Work out the finished part from the listing and answer in its coordinate system (mm). Face numbers are marked on the shaded views. A direction names the side the tool comes from. Give positions to 0.01 mm unless a question says otherwise; leave off trailing zeros. Write each loop counter-clockwise with the first axis right and the second up, starting at its lowest first coordinate (ties: lowest second). Pieces come first, ordered by that corner, then holes. Notation, with made-up numbers: (-14.75, -39) -> (32.25, -39) arc R28 ccw to (32.25, -9) -> close; hole circle Ø11 at (-21, -32). An arc over 180 degrees is marked (long way). Use a Markdown table: item, result. Add a question column.
Q1. Each of these flat-tipped pins is pushed along its axis until it touches: pin 1 Ø2.5 at (y, z) = (0.5, 13) entering from -X; pin 2 Ø7 at (y, z) = (2, 17.5) entering from -X; pin 3 Ø1 at (y, z) = (3.5, 9.5) entering from -X. Where does it stop, or does it pass through?
Q2. Consider line 1 (Y direction, x = -0.75, z = 12.25); line 2 (Y direction, x = -4, z = 10); line 3 (X direction, y = 4.5, z = 23.75). Determine where each line is inside the solid, lowest interval first.
Q3. Section A-A, the plane x = 9.25 is taken. Give the vertices of the cut face in (y, z), plus the area to 3 significant figures.
Q4. Section B-B, the plane z = 5.75 is taken. State how many separate pieces and enclosed holes the cut face has, plus the area to 3 significant figures.
Q5. For a pull along X with two mould halves and no side action, classify the marked faces 1, 2 and 3 as pulls with the +X half, pulls with the -X half, needs draft (parallel to the pull), parting line crosses it, or undercut.
Q6. For the marked faces 4, 5 and 6, determine the directions among +Z, -Z, +X, -X, +Y, -Y from which every point of the face is accessible in a straight line to the end or side of a thin tool.
from build123d import *

# Parameters (mm, degrees)
EXTRUDE1_DEPTH = 25.4


with BuildPart() as part:
    # Sketch1 → Extrude1 (new body)
    with BuildSketch(Plane.XY):
        with BuildLine():
            Line((-8.268033791, 7.446247994), (-5.358427067, 4.536641271))
            ThreePointArc((-5.358427067, 4.536641271), (-4.478329805, 3.219482637), (-4.169280745, 1.665788092))
            Line((-4.169280745, 1.665788092), (-4.169280745, 0))
            Line((-4.169280745, 0), (-4.169280745, -1.665788092))
            ThreePointArc((-4.169280745, -1.665788092), (-4.478329805, -3.219482637), (-5.358427067, -4.536641271))
            Line((-5.358427067, -4.536641271), (-8.268033791, -7.446247994))
            ThreePointArc((-8.268033791, -7.446247994), (-9.379617585, -7.667355758), (-10.009279225, -6.72500052))
            Line((-10.009279225, -6.72500052), (-10.009279225, -4.25999656))
            ThreePointArc((-10.009279225, -4.25999656), (-10.308029711, -3.538749086), (-11.029277185, -3.2399986))
            Line((-11.029277185, -3.2399986), (-11.23000167, -3.2399986))
            ThreePointArc((-11.23000167, -3.2399986), (-11.937549497, -3.525304849), (-12.249277285, -4.221616108))
            Line((-12.249277285, -4.221616108), (-12.49887312, -10.850171322))
            ThreePointArc((-12.49887312, -10.850171322), (-12.055256326, -12.012943733), (-10.90999977, -12.49999913))
            Line((-10.90999977, -12.49999913), (0, -12.49999913))
            Line((0, -12.49999913), (10.90999977, -12.49999913))
            ThreePointArc((10.90999977, -12.49999913), (12.0342991, -12.0342991), (12.49999913, -10.90999977))
            Line((12.49999913, -10.90999977), (12.49999913, 10.90999977))
            ThreePointArc((12.49999913, 10.90999977), (12.0342991, 12.0342991), (10.90999977, 12.49999913))
            Line((10.90999977, 12.49999913), (0, 12.49999913))
            Line((0, 12.49999913), (-10.90999977, 12.49999913))
            ThreePointArc((-10.90999977, 12.49999913), (-12.055256326, 12.012943733), (-12.49887312, 10.850171322))
            Line((-12.49887312, 10.850171322), (-12.249277285, 4.221616108))
            ThreePointArc((-12.249277285, 4.221616108), (-11.937549497, 3.525304849), (-11.23000167, 3.2399986))
            Line((-11.23000167, 3.2399986), (-11.029277185, 3.2399986))
            ThreePointArc((-11.029277185, 3.2399986), (-10.308029711, 3.538749086), (-10.009279225, 4.25999656))
            Line((-10.009279225, 4.25999656), (-10.009279225, 6.72500052))
            ThreePointArc((-10.009279225, 6.72500052), (-9.379617585, 7.667355758), (-8.268033791, 7.446247994))
        make_face()
        with BuildLine():
            Line((-7.539973637, 8.825029193), (-4.084091296, 5.369146852))
            ThreePointArc((-4.084091296, 5.369146852), (-2.766932662, 4.48904959), (-1.213238118, 4.18000053))
            Line((-1.213238118, 4.18000053), (0, 4.18000053))
            Line((0, 4.18000053), (1.439511835, 4.18000053))
            ThreePointArc((1.439511835, 4.18000053), (2.993206379, 4.48904959), (4.310365013, 5.369146852))
            Line((4.310365013, 5.369146852), (7.493110816, 8.551892654))
            ThreePointArc((7.493110816, 8.551892654), (7.679535009, 9.489110364), (6.8850002, 10.02000155))
            Line((6.8850002, 10.02000155), (0, 10.02000155))
            Line((0, 10.02000155), (-7.04499988, 10.02000155))
            ThreePointArc((-7.04499988, 10.02000155), (-7.691714259, 9.587880817), (-7.539973637, 8.825029193))
        make_face(mode=Mode.SUBTRACT)
        with BuildLine():
            Line((0, -10.02000155), (-7.04499988, -10.02000155))
            ThreePointArc((-7.04499988, -10.02000155), (-7.691714259, -9.587880817), (-7.539973637, -8.825029193))
            Line((-7.539973637, -8.825029193), (-4.084091296, -5.369146852))
            ThreePointArc((-4.084091296, -5.369146852), (-2.766932662, -4.48904959), (-1.213238118, -4.18000053))
            Line((-1.213238118, -4.18000053), (0, -4.18000053))
            Line((0, -4.18000053), (1.439511835, -4.18000053))
            ThreePointArc((1.439511835, -4.18000053), (2.993206379, -4.48904959), (4.310365013, -5.369146852))
            Line((4.310365013, -5.369146852), (7.493110816, -8.551892654))
            ThreePointArc((7.493110816, -8.551892654), (7.679535009, -9.489110364), (6.8850002, -10.02000155))
            Line((6.8850002, -10.02000155), (0, -10.02000155))
        make_face(mode=Mode.SUBTRACT)
        with BuildLine():
            Line((8.551892654, 7.493110816), (5.369146852, 4.310365013))
            ThreePointArc((5.369146852, 4.310365013), (4.48904959, 2.993206379), (4.18000053, 1.439511835))
            Line((4.18000053, 1.439511835), (4.18000053, -1.439511835))
            ThreePointArc((4.18000053, -1.439511835), (4.48904959, -2.993206379), (5.369146852, -4.310365013))
            Line((5.369146852, -4.310365013), (8.551892654, -7.493110816))
            ThreePointArc((8.551892654, -7.493110816), (9.489110364, -7.679535009), (10.02000155, -6.8850002))
            Line((10.02000155, -6.8850002), (10.02000155, 6.8850002))
            ThreePointArc((10.02000155, 6.8850002), (9.489110364, 7.679535009), (8.551892654, 7.493110816))
        make_face(mode=Mode.SUBTRACT)
        with BuildLine():
            ThreePointArc((0, 2.55499997), (-1.806657805, 1.806657805), (-2.55499997, 0))
            ThreePointArc((-2.55499997, 0), (-1.806657805, -1.806657805), (0, -2.55499997))
            ThreePointArc((0, -2.55499997), (1.806657805, -1.806657805), (2.55499997, 0))
            ThreePointArc((2.55499997, 0), (1.806657805, 1.806657805), (0, 2.55499997))
        make_face(mode=Mode.SUBTRACT)
    extrude(amount=EXTRUDE1_DEPTH)


solid = part.part
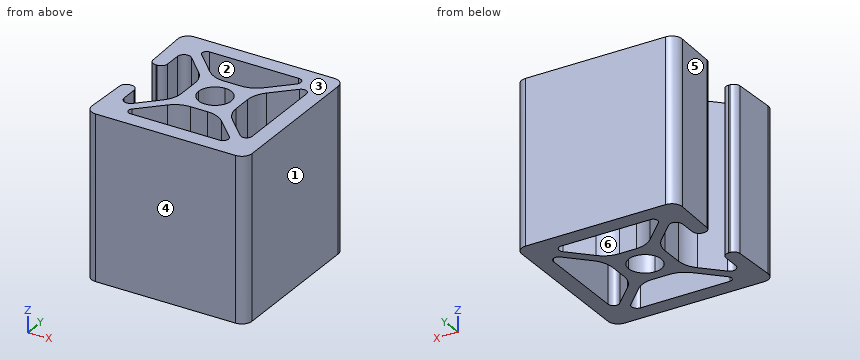
Result set:
| question | item | result |
|---|---|---|
| 1 | pin 1 | stops at x = -4.17 |
| 1 | pin 2 | stops at x = -12.3 |
| 1 | pin 3 | stops at x = -12.22 |
| 2 | line 1 | y = -12.5 to -10.02, -4.18 to -2.44, 2.44 to 4.18, 10.02 to 12.5 |
| 2 | line 2 | y = -12.5 to -10.02, -5.29 to 5.29, 10.02 to 12.5 |
| 2 | line 3 | x = -12.26 to -10.01, -5.32 to -2.79, 3.02 to 5.56, 10.02 to 12.5 |
| 3 | outline | (-12.5, 0) -> (-7.74, 0) -> (-7.74, 25.4) -> (-12.5, 25.4) -> close; (7.74, 0) -> (12.5, 0) -> (12.5, 25.4) -> (7.74, 25.4) -> close |
| 3 | area | 242 mm2 |
| 4 | separate pieces | 1 |
| 4 | enclosed holes | 4 |
| 4 | area | 311 mm2 |
| 5 | face 1 | pulls with the +X half |
| 5 | face 2 | undercut |
| 5 | face 3 | needs draft |
| 6 | face 4 | +Z, -Z, +X, -X, -Y |
| 6 | face 5 | +Z, -Z, -X |
| 6 | face 6 | +Z, -Z |
